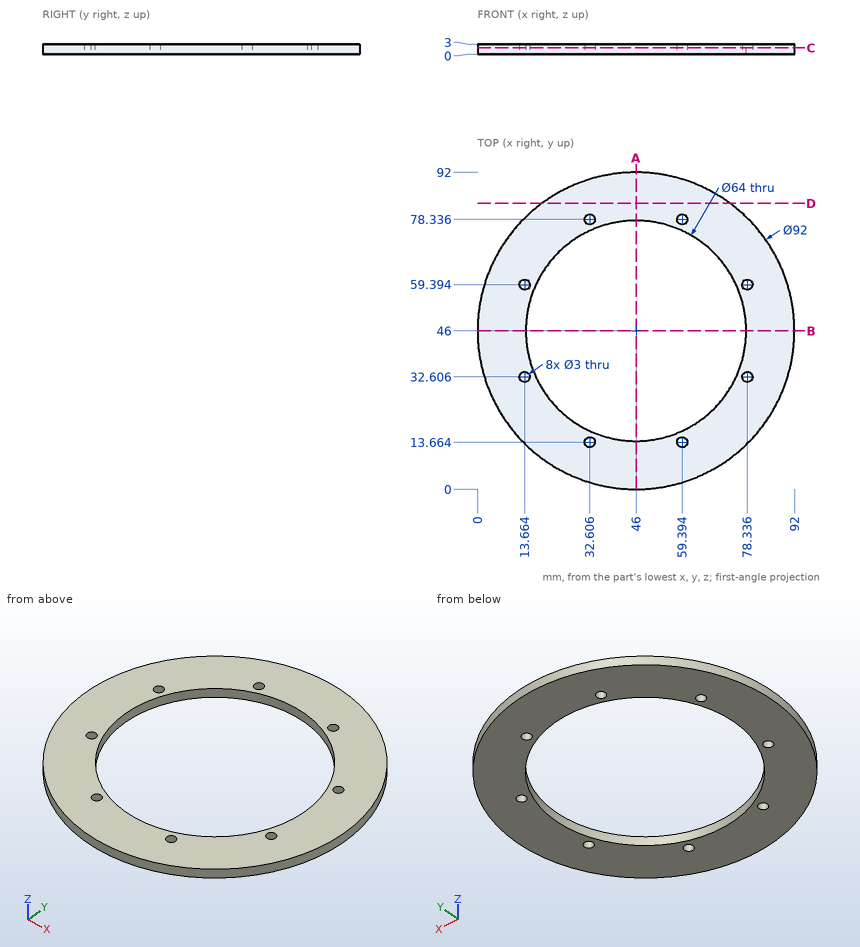
The figure shows three views and two pictorial views of one solid part (mm, origin at its lowest corner). Answer the questions. Give positions to 0.01 mm unless a question says otherwise; leave off trailing zeros. Write each loop counter-clockwise with the first axis right and the second up, starting at its lowest first coordinate (ties: lowest second). Pieces come first, ordered by that corner, then holes. Notation, with made-up numbers: (-28.75, 0) - (5.25, 0) arc R21 cw to (5.25, 14) - close; hole circle Ø3 at (-11.75, 56). An arc over 180 degrees is marked (long way). Use one line per item in the form item = value. Start each with the question number.
1) Find section D-D on y = 83. Determine the outline of the cut face in (x, z).
2) Find section C-C on z = 1.9. Count the separate pieces of the cut face and the enclosed holes in it, plus the area to 3 significant figures.
3) Consider line 1 along X through (y, z) = (59, 2.85) (1 decimal); line 2 along X through (y, z) = (32, 0.8) (1 decimal); line 3 along Y through (x, z) = (36, 1.45). Determine where each line is inside the solid, lowest interval first. Write a range as from..to.
4) Find section A-A on x = 46. Determine the outline of the cut face in (y, z).
Geometry results:
q1.outline = (18.67, 0) - (73.33, 0) - (73.33, 3) - (18.67, 3) - close
q2.separate_pieces = 1
q2.enclosed_holes = 9
q2.area = 3,370 mm2
q3.line_1 = 1.9..12.2, 15.1..16.8, 75.2..76.9, 79.8..90.1
q3.line_2 = 2.2..12.3, 15..17.2, 74.8..77, 79.7..89.8
q3.line_3 = 1.1..15.6, 76.4..90.9
q4.outline = (0, 0) - (14, 0) - (14, 3) - (0, 3) - close; (78, 0) - (92, 0) - (92, 3) - (78, 3) - close
